```python
from build123d import *

# Parameters (mm, degrees)
F0_W     = 15
F0_H     = 20
F0_R     = 2
F1_DEPTH = 3
F2_R     = 3
F3_DEPTH = 3
F5_W     = 30
F5_H     = 3
F6_DEPTH = 6
F7_W     = 2
F7_H     = 2
F8_DEPTH = 30


with BuildPart() as f1:
    # F0 (on Top) → F1 (new body)
    with BuildSketch(Plane.XY):
        with Locations((7.5, -0.262594)):
            Rectangle(F0_W, F0_H)
        with Locations((9, -4.262594)):
            Circle(F0_R, mode=Mode.SUBTRACT)
    extrude(amount=F1_DEPTH)

    # F2 (on face) → F3 (join)
    with BuildSketch(Plane.YZ.offset(15)):
        Polygon((-10.262594, 0), (0, 0), (9.737406, 0), (9.737406, 15), (-10.262594, 3), align=None)
        with BuildLine():
            Line((9.737406, 15), (9.737406, 0))
            Line((9.737406, 0), (40, 0))
            Line((40, 0), (40, 7.5))
            ThreePointArc((40, 7.5), (37.803301, 12.803301), (32.5, 15))
            Line((32.5, 15), (9.737406, 15))
        make_face()
        with Locations((32.5, 7.5)):
            Circle(F2_R, mode=Mode.SUBTRACT)
    extrude(amount=F3_DEPTH)

    # F4: F1 across plane


with BuildPart() as f1_1:
    add(f1.part)
    add(f1.part.mirror(Plane.YZ))

    # F5 (on face) → F6 (join)
    with BuildSketch(Plane.XY.offset(3)):
        with Locations((0, 8.237406)):
            Rectangle(F5_W, F5_H)
    extrude(amount=F6_DEPTH)

    # F7 (on face) → F8 (join, through all)
    with BuildSketch(Plane(origin=(15, 0, 0), x_dir=(0, -1, 0), z_dir=(-1, 0, 0))):
        with Locations((-39, 1)):
            Rectangle(F7_W, F7_H)
    extrude(amount=F8_DEPTH)


solid = f1_1.part
```
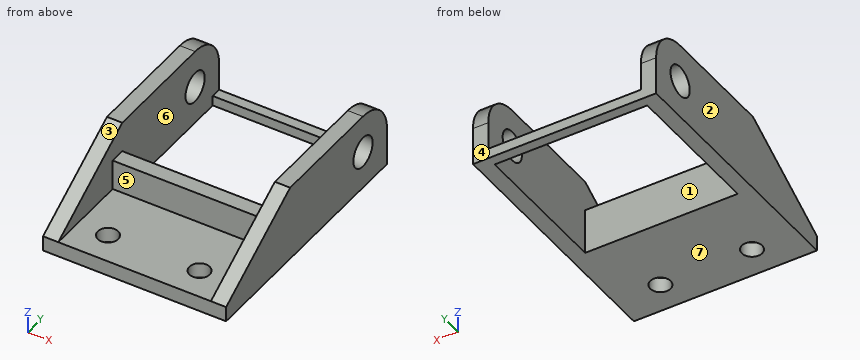
Geometry: final body of the model. Coordinates: model frame, mm. Face numbers are marked on the shaded views. A direction names the side the tool comes from. Give positions to 0.01 mm unless a question says otherwise; leave off trailing zeros. Loops run counter-clockwise (first coordinate to the right, second up) from the corner with the lowest first, then second, coordinate; pieces in that order, holes last. Notation, with made-up numbers: (26.5, -21) - (68.5, -21) arc R29 cw to (68.5, 11) - close; hole circle Ø7 at (80.5, -21.5). An arc over 180 degrees is marked (long way). Answer as CSV lines item,"result". Start each with the question number.
(1) Ray query, line 1 along Y through (x, z) = (9, 0.95); line 2 along X through (y, z) = (18, 11.25); line 3 along Z through (x, y) = (15.85, 32.5). Return the intervals inside material, ascending. Write a range as [from, to].
(2) Section query C-C (x = -4). Output: boundary loops of the cut face in (y, z), and give its area (3 significant figures).
(3) Mould query, pull axis Y, two halves, no side actions, for the marked faces 1, 2, 3 and 4. Classes: +Y half, -Y half, draft (parallel to the pull), parting line (faces both ways), or undercut.
(4) Reachability of the marked faces 5, 6 and 7 from +Z, -Z, +X, -X, +Y, -Y: full face, straight path, thin tool, end or side. Return the list, or none.
(5) Section query A-A (x = -9). Output: boundary loops of the cut face in (y, z).
(6) Pin query (flat end, axial travel): P1, Ø7, axis at y = 32.5, z = 7.5, coming from the -X side; P2, Ø0.6, axis at x = 3.5, y = 39, coming from the +Z side; P3, Ø3.5, axis at x = 0, y = 7.5, coming from the +Z side; P4, Ø4.5, axis at x = 1.5, z = 6, coming from the +Y side. Return the tip coordinate at first contact, or that it passes through.
(7) Section query B-B (y = 16.5). Output: boundary loops of the cut face in (x, z).
(8) Section query D-D (z = 13.75). Output: boundary loops of the cut face in (x, y), and give its area (3 significant figures).
Worked answers:
1,line 1,"y = [-10.26, -6.26], [-2.26, 9.74], [38, 40]"
1,line 2,"x = [-18, -15], [15, 18]"
1,line 3,"z = [0, 4.5], [10.5, 15]"
2,outline,"(-10.26, 0) - (9.74, 0) - (9.74, 9) - (6.74, 9) - (6.74, 3) - (-10.26, 3) - close; (38, 0) - (40, 0) - (40, 2) - (38, 2) - close"
2,area,"82.0 mm^2"
3,face 1,"undercut"
3,face 2,"draft"
3,face 3,"-Y half"
3,face 4,"+Y half"
4,face 5,"+Z, -Y"
4,face 6,"+Z"
4,face 7,"-Z, +X, -X, +Y, -Y"
5,outline,"(-10.26, 0) - (-6.26, 0) - (-6.26, 3) - (-10.26, 3) - close; (-2.26, 0) - (9.74, 0) - (9.74, 9) - (6.74, 9) - (6.74, 3) - (-2.26, 3) - close; (38, 0) - (40, 0) - (40, 2) - (38, 2) - close"
6,P1,"stops at x = -18"
6,P2,"stops at z = 2"
6,P3,"stops at z = 9"
6,P4,"stops at y = 9.74"
7,outline,"(-18, 0) - (-15, 0) - (-15, 15) - (-18, 15) - close; (15, 0) - (18, 0) - (18, 15) - (15, 15) - close"
8,outline,"(-18, 7.65) - (-15, 7.65) - (-15, 36.65) - (-18, 36.65) - close; (15, 7.65) - (18, 7.65) - (18, 36.65) - (15, 36.65) - close"
8,area,"174 mm^2"
